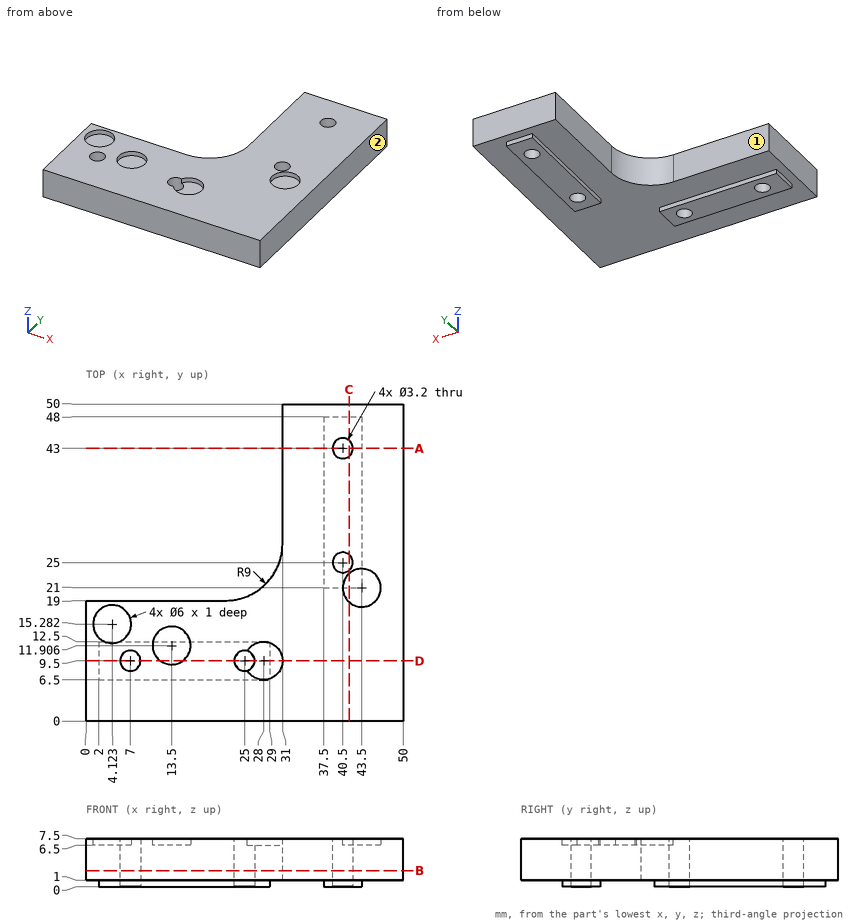
Here's the drawing with two shaded views (mm, measured from the low corner). I have some questions. A direction names the side the tool comes from. Round coordinates to 2 decimals unless told otherwise and drop trailing zeros. Write each loop counter-clockwise with the first axis right and the second up, starting at its lowest first coordinate (ties: lowest second). Pieces come first, ordered by that corner, then holes. Notation, with made-up numbers: M -16.5,0.5 L -8.5,0.5 A30 ccw -8.5,32.5 Z; hole C -6,2.5 d9. An arc over 180 degrees is marked long. Answer in a Markdown table with one row per item. Add a question column.
Q1. Imagine slicing it at B-B (z = 2.5). Please give me the cut outline in (x, y).
Q2. If I drill on line 1 (Y direction, x = 43.5, z = 6.85); line 2 (Y direction, x = 7, z = 5.5); line 3 (X direction, y = 10.5, z = 3.5), over which ranges is the centre line in solid material (lowest first)? Write a range as from..to.
Q3. On a 3-axis mill with a long thin cutter (end or side, diameter ignored), from which of +Z, -Z, +X, -X, +Y, -Y can I reach the whole of each face in a straight line? I mean the marked faces 1 and 2. Say none if no direction works.
Q4. Will these pins go through, and if not, where does the flat tip stop? pin 1 Ø0.5 at (x, z) = (19.5, 0.5) entering from -Y; pin 2 Ø5 at (x, y) = (43.5, 21) entering from +Z; pin 3 Ø0.8 at (x, z) = (14, 0.5) entering from +Y.
Q5. Imagine slicing it at A-A (y = 43). Please give me the cut outline in (x, z), then the cut area to 4 significant figures.
Q6. Imagine slicing it at C-C (x = 41.5). Please give me the cut outline in (y, z).
Q7. Imagine slicing it at D-D (y = 9.5). Please give me the cut outline in (x, z).
Values:
| question | item | result |
|---|---|---|
| 1 | outline | M 0,0 L 50,0 L 50,50 L 31,50 L 31,28 A9 cw 22,19 L 0,19 Z; hole C 7,9.5 d3.2; hole C 25,9.5 d3.2; hole C 40.5,25 d3.2; hole C 40.5,43 d3.2 |
| 2 | line 1 | 0..18, 24..50 |
| 2 | line 2 | 0..7.9, 11.1..19 |
| 2 | line 3 | 0..5.75, 8.25..23.75, 26.25..50 |
| 3 | face 1 | +Z, -Z, -X, +Y |
| 3 | face 2 | +Z, -Z, +X, +Y, -Y |
| 4 | pin 1 | y = 6.5 |
| 4 | pin 2 | z = 6.5 |
| 4 | pin 3 | y = 12.5 |
| 5 | outline | M 31,1 L 37.5,1 L 37.5,0 L 38.9,0 L 38.9,7.5 L 31,7.5 Z; M 42.1,0 L 43.5,0 L 43.5,1 L 50,1 L 50,7.5 L 42.1,7.5 Z |
| 5 | area | 105.5 mm^2 |
| 6 | outline | M 0,1 L 21,1 L 21,0 L 23.75,0 L 23.75,7.5 L 23.24,7.5 L 23.24,6.5 L 18.76,6.5 L 18.76,7.5 L 0,7.5 Z; M 26.25,0 L 41.75,0 L 41.75,7.5 L 26.25,7.5 Z; M 44.25,0 L 48,0 L 48,1 L 50,1 L 50,7.5 L 44.25,7.5 Z |
| 7 | outline | M 0,1 L 2,1 L 2,0 L 5.4,0 L 5.4,7.5 L 0,7.5 Z; M 8.6,0 L 23.4,0 L 23.4,7.5 L 15.29,7.5 L 15.29,6.5 L 11.71,6.5 L 11.71,7.5 L 8.6,7.5 Z; M 26.6,0 L 29,0 L 29,1 L 50,1 L 50,7.5 L 31,7.5 L 31,6.5 L 26.6,6.5 Z |
